Job drawing, mm, ordinate dimensions from the low corner. One solid piece. Round coordinates to 2 decimals unless told otherwise and drop trailing zeros. Order: outer loops, then holes, each group sorted by start corner. A loop starts at its lowest first (then second) coordinate and runs counter-clockwise, first axis right, second up. Notation, with made-up numbers: (18.25, -24.5) -> (24.25, -24.5) arc R36 ccw to (24.25, 9.5) -> close; hole circle Ø1 at (-38.75, 53). An arc over 180 degrees is marked (long way). Answer as a JSON object with one key per item and string values. Group by question number.
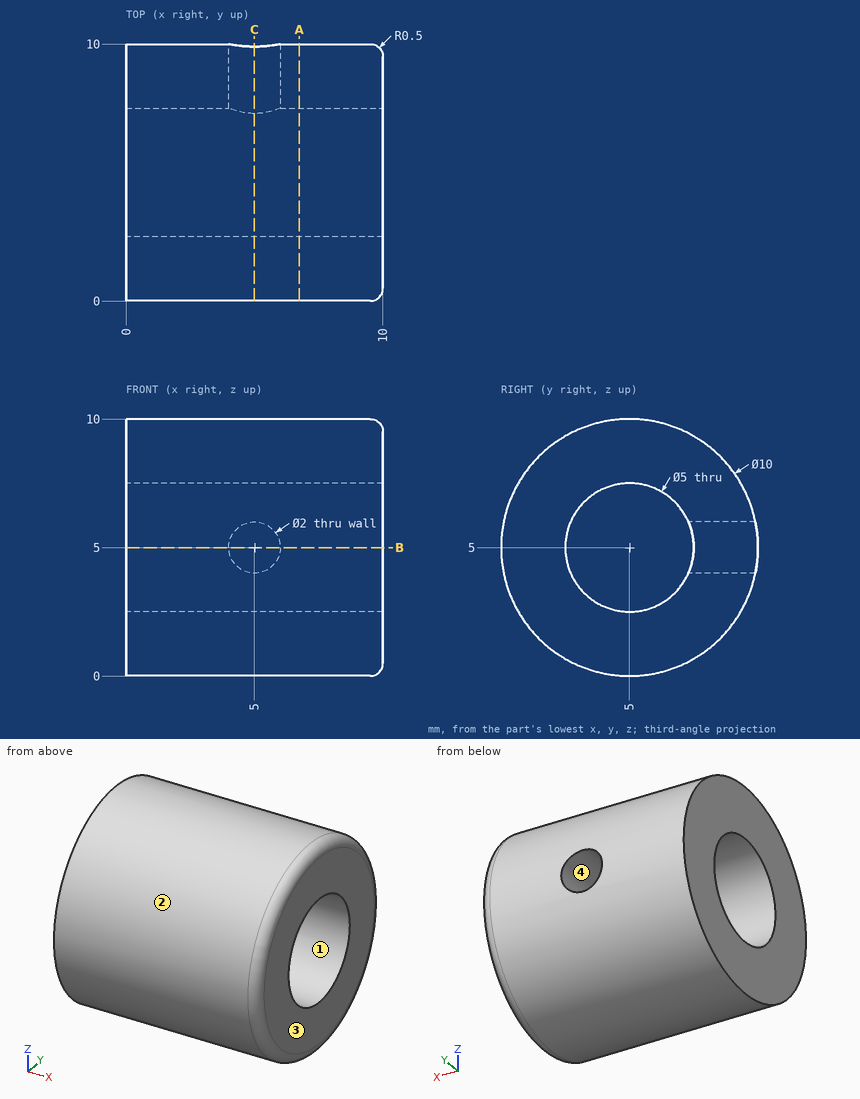
Q1. Drop flat-ended pins along their axis: pin 1 Ø1.5 at (x, z) = (1.5, 1.5) entering from +Y; pin 2 Ø1 at (x, z) = (6.5, 8) entering from -Y. Give the stop position or say it passes through.
Q2. Band-saw the part on A-A (x = 6.75). List the corners of the cut face in (y, z).
Q3. Two-plate mould, pull along Z, no slides. Class the marked faces 1, 2, 3 and 4: +Z half, -Z half, draft (parallel to the pull), parting line (faces both ways), or undercut.
Q4. Band-saw the part on C-C (x = 5). List the corners of the cut face in (y, z).
Q5. Wall check: line 1 (Z direction, x = 2, y = 5); line 2 (Z direction, x = 5, y = 7.9); line 3 (Y direction, x = 1.75, z = 3). Give the ranges that are in metal, low to high. Write a range as [from, to].
Q6. Band-saw the part on B-B (z = 5). Count the separate pieces of the cut face and the enclosed holes in it, plus the area to 3 significant figures.
Completed:
{
 "1": {"pin 1": "y = 9.18", "pin 2": "y = 0.67"},
 "2": {"outline": "circle Ø10 at (5, 5); hole circle Ø5 at (5, 5)"},
 "3": {"face 1": "undercut", "face 2": "parting line", "face 3": "draft", "face 4": "undercut"},
 "4": {"outline": "(7.29, 4) arc R2.5 cw (long way) to (7.29, 6) -> (9.9, 6) arc R5 ccw (long way) to (9.9, 4) -> close"},
 "5": {"line 1": "[0, 2.5], [7.5, 10]", "line 2": "[0.93, 4], [6, 9.07]", "line 3": "[0.42, 3.5], [6.5, 9.58]"},
 "6": {"separate pieces": "3", "enclosed holes": "0", "area": "44.9 mm2"}
}
